Answer from the drawing. Dimensions are ordinates in mm from the lowest x, y and z of the part. Round coordinates to 2 decimals unless told otherwise and drop trailing zeros. Write each loop counter-clockwise with the first axis right and the second up, starting at its lowest first coordinate (ties: lowest second). Pieces come first, ordered by that corner, then holes. Notation, with made-up numbers: (23, -6.75) -> (60, -6.75) arc R18 cw to (60, 21.25) -> close; hole circle Ø4 at (22.25, 2). An arc over 180 degrees is marked (long way). Return JSON: item names as keys, results as strings. Group by question number.
(1) A cutting plane is placed at A-A on y = 12.7. Give the vertices of the cut face in (x, z), then the cut area to 3 significant figures.
(2) A cutting plane is placed at C-C on z = 3.5. Give the vertices of the cut face in (x, y).
(3) The mould has two halves that part along Y. Classify the marked faces 1, 2 and 3: released by +Y, released by -Y, zero draft, split by the parting line, or undercut.
(4) A cutting plane is placed at D-D on y = 8. Give the vertices of the cut face in (x, z), then the cut area to 3 significant figures.
(5) A cutting plane is placed at B-B on x = 27.94. Give the vertices of the cut face in (y, z), then the cut area to 3 significant figures.
(6) Straight lines are drawn through the part: line 1 (Y direction, x = 27.94, z = 1.75); line 2 (Y direction, x = 49.13, z = 3); line 3 (X direction, y = 13.5, z = 1.75). For each, find the intervals that lie inside material, in ascending order.
(7) Given pin 1 (3 mm diameter, centred on x = 49.13, y = 12.7, fed in from -Z); pin 2 (3 mm diameter, centred on y = 23, z = 2.5, fed in from +X), each flat-ended and moving along its own axis, determine where each tip first touches the part or whether it passes through.
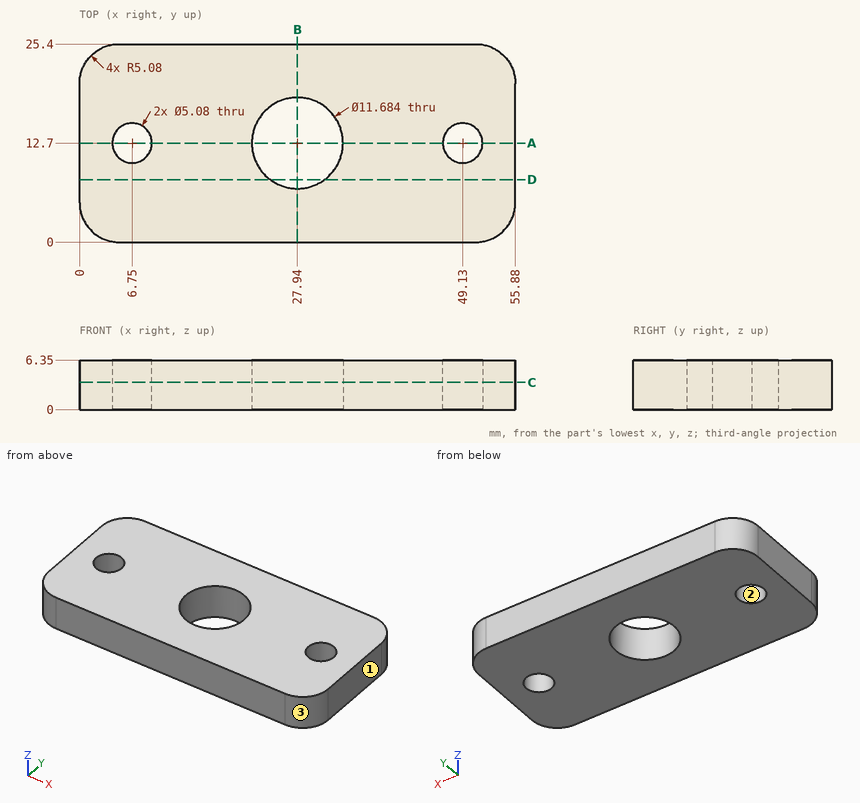
Checks:
{
 "1": {"outline": "(0, 0) -> (4.21, 0) -> (4.21, 6.35) -> (0, 6.35) -> close; (9.29, 0) -> (22.1, 0) -> (22.1, 6.35) -> (9.29, 6.35) -> close; (33.78, 0) -> (46.59, 0) -> (46.59, 6.35) -> (33.78, 6.35) -> close; (51.67, 0) -> (55.88, 0) -> (55.88, 6.35) -> (51.67, 6.35) -> close", "area": "216 mm^2"},
 "2": {"outline": "(0, 5.08) arc R5.08 ccw to (5.08, 0) -> (50.8, 0) arc R5.08 ccw to (55.88, 5.08) -> (55.88, 20.32) arc R5.08 ccw to (50.8, 25.4) -> (5.08, 25.4) arc R5.08 ccw to (0, 20.32) -> close; hole circle Ø5.08 at (6.75, 12.7); hole circle Ø11.68 at (27.94, 12.7); hole circle Ø5.08 at (49.13, 12.7)"},
 "3": {"face 1": "zero draft", "face 2": "undercut", "face 3": "released by -Y"},
 "4": {"outline": "(0, 0) -> (24.47, 0) -> (24.47, 6.35) -> (0, 6.35) -> close; (31.41, 0) -> (55.88, 0) -> (55.88, 6.35) -> (31.41, 6.35) -> close", "area": "311 mm^2"},
 "5": {"outline": "(0, 0) -> (6.86, 0) -> (6.86, 6.35) -> (0, 6.35) -> close; (18.54, 0) -> (25.4, 0) -> (25.4, 6.35) -> (18.54, 6.35) -> close", "area": "87.1 mm^2"},
 "6": {"line 1": "y = 0 to 6.86, 18.54 to 25.4", "line 2": "y = 0 to 10.16, 15.24 to 25.4", "line 3": "x = 0 to 4.34, 9.16 to 22.15, 33.73 to 46.72, 51.54 to 55.88"},
 "7": {"pin 1": "passes through", "pin 2": "stops at x = 55.74"}
}
